Input: dimensioned drawing with shaded views. Units: mm. Origin: part minimum x, y, z. Coordinates: 2 decimals unless noted, no trailing zeros. Order: outer loops, then holes, each group sorted by start corner. A loop starts at its lowest first (then second) coordinate and runs counter-clockwise, first axis right, second up.
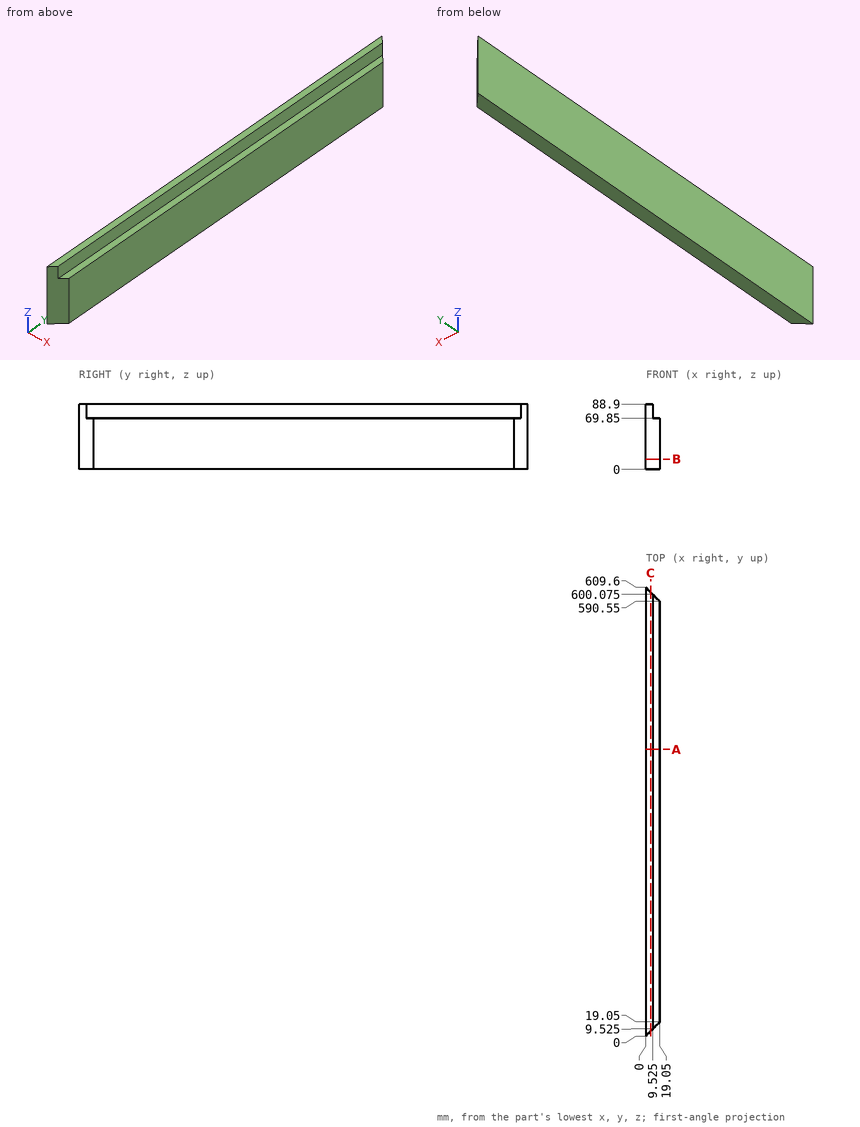
1. Section query C-C on x = 6.5. Return loops of the section in (y, z).
Findings:
outline: (6.5, 0) - (603.1, 0) - (603.1, 88.9) - (6.5, 88.9) - close
2. Section query A-A on y = 389.5. Return loops of the section in (x, z) (3 decimals).
Findings:
outline: (0, 0) - (19.05, 0) - (19.05, 69.85) - (9.525, 69.85) - (9.525, 88.9) - (0, 88.9) - close
3. Section query B-B on z = 14. Return loops of the section in (x, y).
Findings:
outline: (0, 0) - (19.05, 19.05) - (19.05, 590.55) - (0, 609.6) - close
4. Pin query (flat end, axial travel): P1, Ø1.5, axis at x = 11, y = 76, coming from the +Z side; P2, Ø10, axis at x = 15, z = 57, coming from the +Y side; P3, Ø4, axis at x = 15.5, z = 10, coming from the +Y side. Return the tip coordinate at first contact, or that it passes through.
Findings:
P1: stops at z = 69.85
P2: stops at y = 599.6
P3: stops at y = 596.1
5. Ray query, line 1 (X direction, y = 305, z = 85) (3 decimals); line 2 (Z direction, x = 13.25, y = 301.5); line 3 (Y direction, x = 5.5, z = 80). Return the intervals inside material, ascending.
Findings:
line 1: x = 0 to 9.525
line 2: z = 0 to 69.85
line 3: y = 5.5 to 604.1
